Input: dimensioned drawing with shaded views. Units: mm. Origin: part minimum x, y, z. Give positions to 0.01 mm unless a question says otherwise; leave off trailing zeros. Order: outer loops, then holes, each group sorted by start corner. A loop starts at its lowest first (then second) coordinate and runs counter-clockwise, first axis right, second up. Notation, with made-up numbers: (63, 43.25) - (90, 43.25) arc R11 ccw to (90, 57.25) - close; hole circle Ø2 at (81, 1). An arc over 180 degrees is marked (long way). Answer as CSV lines item,"result".
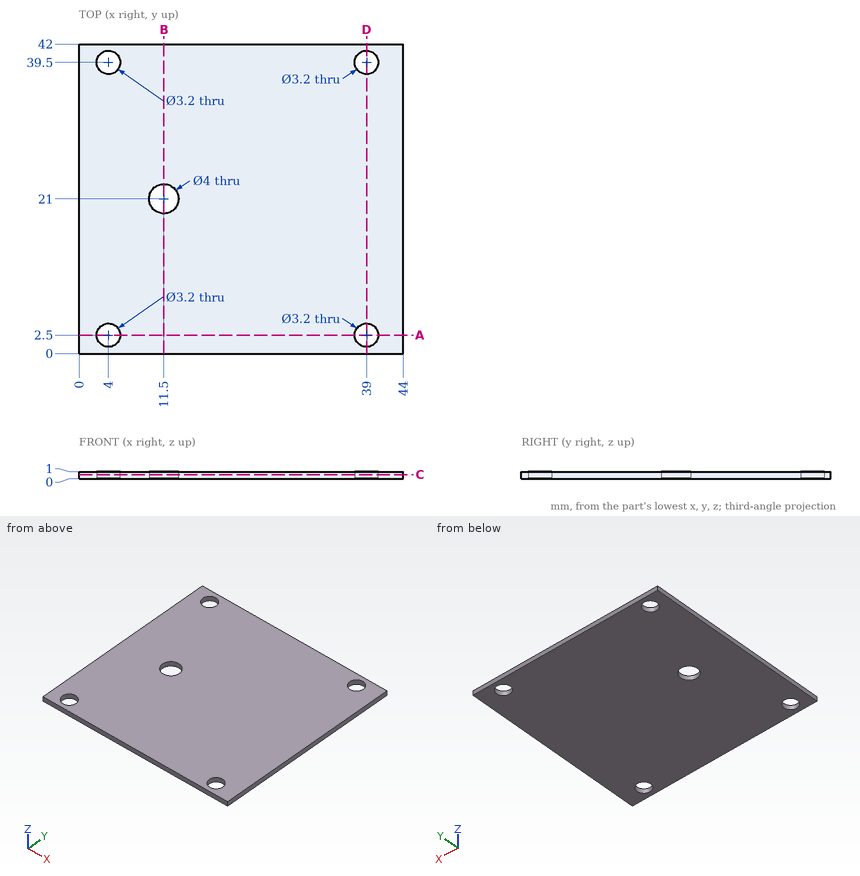
(1) Cut plane A-A (y = 2.5). Return loops of the section in (x, z).
Completed:
outline,"(0, 0) - (2.4, 0) - (2.4, 1) - (0, 1) - close; (5.6, 0) - (37.4, 0) - (37.4, 1) - (5.6, 1) - close; (40.6, 0) - (44, 0) - (44, 1) - (40.6, 1) - close"
(2) Contact query for a flat-ended pin moving along its axis: pin 1 (3 mm diameter, centred on x = 4, y = 39.5, fed in from +Z). Output: stop coordinate, or through.
Completed:
pin 1,"through"
(3) Cut plane D-D (x = 39). Return loops of the section in (y, z), then the cut area to 3 significant figures.
Completed:
outline,"(0, 0) - (0.9, 0) - (0.9, 1) - (0, 1) - close; (4.1, 0) - (37.9, 0) - (37.9, 1) - (4.1, 1) - close; (41.1, 0) - (42, 0) - (42, 1) - (41.1, 1) - close"
area,"35.6 mm²"
(4) Cut plane B-B (x = 11.5). Return loops of the section in (y, z).
Completed:
outline,"(0, 0) - (19, 0) - (19, 1) - (0, 1) - close; (23, 0) - (42, 0) - (42, 1) - (23, 1) - close"
(5) Cut plane C-C (z = 0.6). Return loops of the section in (x, y), then the cut area to 3 significant figures.
Completed:
outline,"(0, 0) - (44, 0) - (44, 42) - (0, 42) - close; hole circle Ø3.2 at (4, 2.5); hole circle Ø3.2 at (4, 39.5); hole circle Ø4 at (11.5, 21); hole circle Ø3.2 at (39, 2.5); hole circle Ø3.2 at (39, 39.5)"
area,"1,800 mm²"
(6) Ray query, line 1 (Y direction, x = 39, z = 0.3); line 2 (X direction, y = 39.5, z = 0.45); line 3 (X direction, y = 21, z = 0.35). Return the intervals inside material, ascending. Write a range as from..to.
Completed:
line 1,"0..0.9, 4.1..37.9, 41.1..42"
line 2,"0..2.4, 5.6..37.4, 40.6..44"
line 3,"0..9.5, 13.5..44"
